Part model, mm, in its own coordinate system. Face numbers are marked on the shaded views. A direction names the side the tool comes from. Give positions to 0.01 mm unless a question says otherwise; leave off trailing zeros. Write each loop counter-clockwise with the first axis right and the second up, starting at its lowest first coordinate (ties: lowest second). Pieces come first, ordered by that corner, then holes. Notation, with made-up numbers: (-16.75, -14.5) - (30.25, -14.5) arc R4 ccw to (30.25, -7.5) - close; hole circle Ø7 at (-40, 28.25). An arc over 180 degrees is marked (long way). Answer in a Markdown table with one row per item. Add a question column.
1. Drop flat-ended pins along their axis: pin 1 Ø1.9 at (y, z) = (7.5, 1) entering from +X; pin 2 Ø4 at (y, z) = (-8.5, -30.5) entering from -X; pin 3 Ø4 at (x, z) = (11.43, -54.61) entering from +Y; pin 4 Ø6 at (x, y) = (23.5, -7.5) entering from +Z (3 decimals). Give the stop position or say it passes through.
2. Band-saw the part on B-B on z = -17.5. Write the cut outline in (x, y).
3. Probe line 1 along X through (y, z) = (2, -3.81); line 2 along X through (y, z) = (7.2, -54.61); line 3 along Z through (x, y) = (11, 3) (3 decimals). List the from-to ranges inside material, lowest first.
4. Which spindle directions (+Z, -Z, +X, -X, +Y, -Y) get a long thin tool onto all of the face, cutting with end or side? Do the marked faces 5, 6, 7, 8 and 9. Say none if no direction does.
5. Band-saw the part on D-D on x = 22. Write the cut outline in (y, z) (3 decimals).
6. Band-saw the part on A-A on x = 11.43. Write the cut outline in (y, z) (3 decimals), plus the area to 3 significant figures.
7. Pull direction Z, two halves, no side cores. Call the marked faces 1, 2, 3 and 4: released by +Z, released by -Z, zero draft, split by the parting line, or undercut.
8. Band-saw the part on C-C on y = -10.5. Write the cut outline in (x, z) (3 decimals).
```python
from build123d import *

# Parameters (mm, degrees)
SKETCH1_R           = 3.302
SKETCH1_R_2         = 2.615549664
BOSS_EXTRUDE1_DEPTH = 6.35
SKETCH2_W           = 30.48
SKETCH2_H           = 50.8
CUT_EXTRUDE1_DEPTH  = 3.81
CUT_EXTRUDE2_DEPTH  = 83.161835082
SKETCH13_R          = 2.615549664
BOSS_EXTRUDE7_DEPTH = 3.81
SKETCH15_W          = 7.62
SKETCH15_H          = 44.704
BOSS_EXTRUDE8_DEPTH = 21.59
SKETCH16_R          = 1.27
CUT_EXTRUDE3_DEPTH  = 81.375650193
FILLET1_R           = 2.54
CHAMFER2_SIZE       = 2.54


with BuildPart() as part:
    # Sketch1 → Boss-Extrude1 (new body)
    with BuildSketch(Plane(origin=(0, 0, 0), x_dir=(1, 0, 0), z_dir=(0, 1, 0))):
        Polygon((50.8, -0.508), (25.4, -5.588), (-25.4, -5.588), (-25.4, 64.262), (25.4, 64.262), (50.8, 59.182), align=None)
        with Locations(Location((0, 0, 0), (0, 0, 270))):
            Circle(SKETCH1_R, mode=Mode.SUBTRACT)
        with Locations(Location((0, 58.674, 0), (0, 0, 270))):
            Circle(SKETCH1_R, mode=Mode.SUBTRACT)
        with Locations(Location((11.43, 54.61, 0), (0, 0, 270))):
            Circle(SKETCH1_R_2, mode=Mode.SUBTRACT)
        with Locations(Location((-20.32, 54.61, 0), (0, 0, 270))):
            Circle(SKETCH1_R_2, mode=Mode.SUBTRACT)
        with Locations(Location((-20.32, 3.81, 0), (0, 0, 270))):
            Circle(SKETCH1_R_2, mode=Mode.SUBTRACT)
        with Locations(Location((11.43, 3.81, 0), (0, 0, 270))):
            Circle(SKETCH1_R_2, mode=Mode.SUBTRACT)
    extrude(amount=BOSS_EXTRUDE1_DEPTH)

    # Sketch2 → Cut-Extrude1 (cut)
    with BuildSketch(Plane(origin=(0, 6.35, 0), x_dir=(1, 0, 0), z_dir=(0, 1, 0))):
        with Locations((33.02, 29.337)):
            Rectangle(SKETCH2_W, SKETCH2_H)
    extrude(amount=-CUT_EXTRUDE1_DEPTH, mode=Mode.SUBTRACT)

    # Sketch3 → Cut-Extrude2 (cut, through all)
    with BuildSketch(Plane(origin=(0, 6.35, 0), x_dir=(1, 0, 0), z_dir=(0, 1, 0))):
        with BuildLine():
            Line((-15.24, 58.674), (-15.24, 51.689))
            Line((-15.24, 51.689), (5.08, 51.689))
            Line((5.08, 51.689), (5.08, 58.674))
            Line((5.08, 58.674), (3.302, 58.674))
            ThreePointArc((3.302, 58.674), (0, 55.372), (-3.302, 58.674))
            Line((-3.302, 58.674), (-15.24, 58.674))
        make_face()
        Polygon((-15.24, 51.689), (-25.4, 51.689), (-25.4, 6.985), (-15.24, 6.985), (5.08, 6.985), (17.78, 6.985), (17.78, 51.689), (5.08, 51.689), align=None)
        with BuildLine():
            Line((5.08, 6.985), (-15.24, 6.985))
            Line((-15.24, 6.985), (-15.24, 0))
            Line((-15.24, 0), (-3.302, 0))
            ThreePointArc((-3.302, 0), (0, 3.302), (3.302, 0))
            Line((3.302, 0), (5.08, 0))
            Line((5.08, 0), (5.08, 6.985))
        make_face()
    extrude(amount=-CUT_EXTRUDE2_DEPTH, mode=Mode.SUBTRACT)

    # Sketch13 → Boss-Extrude7 (add)
    # profile 1 of 2: a face of its own
    with BuildSketch(Plane(origin=(0, 6.35, 0), x_dir=(1, 0, 0), z_dir=(0, 1, 0))):
        with BuildLine():
            Line((-25.4, 64.262), (-25.4, 51.689))
            Line((-25.4, 51.689), (-15.24, 51.689))
            Line((-15.24, 51.689), (-15.24, 58.674))
            Line((-15.24, 58.674), (-3.302, 58.674))
            ThreePointArc((-3.302, 58.674), (0, 61.976), (3.302, 58.674))
            Line((3.302, 58.674), (5.08, 58.674))
            Line((5.08, 58.674), (5.08, 51.689))
            Line((5.08, 51.689), (17.78, 51.689))
            Line((17.78, 51.689), (17.78, 54.737))
            Line((17.78, 54.737), (25.4, 54.737))
            Line((25.4, 54.737), (25.4, 64.262))
            Line((25.4, 64.262), (-25.4, 64.262))
        make_face()
        with Locations(Location((-20.32, 54.61, 0), (0, 0, 270))):
            Circle(SKETCH13_R, mode=Mode.SUBTRACT)
        with Locations(Location((11.43, 54.61, 0), (0, 0, 270))):
            Circle(SKETCH13_R, mode=Mode.SUBTRACT)
    # profile 2 of 2: a face of its own
    with BuildSketch(Plane(origin=(0, 6.35, 0), x_dir=(1, 0, 0), z_dir=(0, 1, 0))):
        with BuildLine():
            Line((-15.24, 6.985), (-25.4, 6.985))
            Line((-25.4, 6.985), (-25.4, -5.588))
            Line((-25.4, -5.588), (25.4, -5.588))
            Line((25.4, -5.588), (25.4, 3.937))
            Line((25.4, 3.937), (17.78, 3.937))
            Line((17.78, 3.937), (17.78, 6.985))
            Line((17.78, 6.985), (5.08, 6.985))
            Line((5.08, 6.985), (5.08, 0))
            Line((5.08, 0), (3.302, 0))
            ThreePointArc((3.302, 0), (0, -3.302), (-3.302, 0))
            Line((-3.302, 0), (-15.24, 0))
            Line((-15.24, 0), (-15.24, 6.985))
        make_face()
        with Locations(Location((-20.32, 3.81, 0), (0, 0, 270))):
            Circle(SKETCH13_R, mode=Mode.SUBTRACT)
        with Locations(Location((11.43, 3.81, 0), (0, 0, 270))):
            Circle(SKETCH13_R, mode=Mode.SUBTRACT)
    extrude(amount=BOSS_EXTRUDE7_DEPTH)

    # Sketch15 → Boss-Extrude8 (add)
    with BuildSketch(Plane.XZ):
        with Locations((21.59, -29.337)):
            Rectangle(SKETCH15_W, SKETCH15_H)
    extrude(amount=BOSS_EXTRUDE8_DEPTH)

    # Sketch16 → Cut-Extrude3 (cut, through all)
    with BuildSketch(Plane.ZY.offset(-17.78)):
        with Locations((-44.323, -18.542)):
            Circle(SKETCH16_R)
        with Locations((-34.671, -18.542)):
            Circle(SKETCH16_R)
        with Locations((-24.003, -18.542)):
            Circle(SKETCH16_R)
        with Locations((-14.351, -18.542)):
            Circle(SKETCH16_R)
    extrude(amount=-CUT_EXTRUDE3_DEPTH, mode=Mode.SUBTRACT)

    # Fillet1
    # the kernel refuses this fillet: 2.54 mm, written as the material it adds along each edge
    with BuildSketch(Plane(origin=(-15.24, 0, -58.674), x_dir=(0, 0, 1), z_dir=(0, 1, 0))) as fillet1_piece_1:
        with BuildLine():
            CenterArc((FILLET1_R, FILLET1_R), FILLET1_R, 180, 90)
            Line((0, FILLET1_R), (0, 0))
            Line((0, 0), (FILLET1_R, 0))
        make_face()
    extrude(amount=10.16)
    with BuildSketch(Plane(origin=(5.08, 10.16, -58.674), x_dir=(-1, 0, 0), z_dir=(0, -1, 0))) as fillet1_piece_2:
        with BuildLine():
            CenterArc((2.54, -2.423005572), FILLET1_R, 107.457603124, 72.542396876)
            Line((0, -2.423005572), (0, 0))
            Line((0, 0), (1.778, 0))
        make_face()
    extrude(amount=10.16)
    with BuildSketch(Plane(origin=(5.08, 10.16, 0), x_dir=(0, 0, -1), z_dir=(0, -1, 0))) as fillet1_piece_3:
        with BuildLine():
            CenterArc((2.423005572, -2.54), FILLET1_R, 90, 72.542396876)
            Line((0, -1.778), (0, 0))
            Line((0, 0), (2.423005572, 0))
        make_face()
    extrude(amount=10.16)
    with BuildSketch(Plane(origin=(-15.24, 10.16, 0), x_dir=(1, 0, 0), z_dir=(0, -1, 0))) as fillet1_piece_4:
        with BuildLine():
            CenterArc((FILLET1_R, -FILLET1_R), FILLET1_R, 90, 90)
            Line((0, -FILLET1_R), (0, 0))
            Line((0, 0), (FILLET1_R, 0))
        make_face()
    extrude(amount=10.16)
    # the kernel refuses this fillet: 2.54 mm, written as the material it takes off along each edge
    with BuildSketch(Plane(origin=(-15.24, -6.35, -51.689), x_dir=(-1, 0, 0), z_dir=(0, 1, 0))) as fillet1_2_piece_1:
        with BuildLine():
            CenterArc((FILLET1_R, -FILLET1_R), FILLET1_R, 90, 90)
            Line((0, -FILLET1_R), (0, 0))
            Line((0, 0), (FILLET1_R, 0))
        make_face()
    extrude(amount=22.86, mode=Mode.SUBTRACT)
    with BuildSketch(Plane(origin=(5.08, 16.51, -51.689), x_dir=(0, 0, -1), z_dir=(0, -1, 0)), Plane(origin=(5.08, 16.51, -6.985), x_dir=(1, 0, 0), z_dir=(0, -1, 0)), Plane(origin=(-15.24, 16.51, -6.985), x_dir=(0, 0, 1), z_dir=(0, -1, 0))) as fillet1_2_piece_2:
        with BuildLine():
            CenterArc((FILLET1_R, FILLET1_R), FILLET1_R, 180, 90)
            Line((0, FILLET1_R), (0, 0))
            Line((0, 0), (FILLET1_R, 0))
        make_face()
    extrude(amount=22.86, mode=Mode.SUBTRACT)

    # Chamfer2
    chamfer2_edges = [part.edges().sort_by_distance(p)[0] for p in [
        (21.59, 0, -51.689),
        (25.4, 0, -29.337),
        (21.59, 0, -6.985),
    ]]
    chamfer(chamfer2_edges, length=CHAMFER2_SIZE)


solid = part.part
```
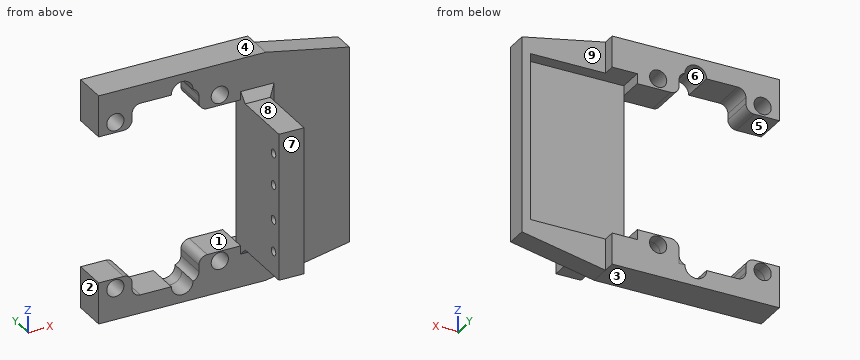
Values:
| question | item | result |
|---|---|---|
| 1 | pin 1 | stops at x = 25.4 |
| 1 | pin 2 | stops at x = 17.78 |
| 1 | pin 3 | passes through |
| 1 | pin 4 | stops at z = -6.985 |
| 2 | outline | (17.78, -21.59) - (25.4, -21.59) - (25.4, -2.54) - (27.94, 0) - (50.8, 0) - (50.8, 6.35) - (48.26, 6.35) - (48.26, 2.54) - (17.78, 2.54) - close |
| 3 | line 1 | x = -25.4 to -22.94, -17.7 to -15.24, 5.08 to 8.81, 14.05 to 50.8 |
| 3 | line 2 | x = -25.4 to -22.94, -17.7 to -15.24, 5.08 to 8.81, 14.05 to 17.78 |
| 3 | line 3 | z = -64.262 to -57.19, -52.03 to -51.689, -6.985 to -6.39, -1.23 to 5.588 |
| 4 | face 5 | -X, +Y, -Y |
| 4 | face 6 | +Y, -Y |
| 4 | face 7 | +Z, -Z, +X, -X, -Y |
| 4 | face 8 | +Z, +X, -X, -Y |
| 4 | face 9 | +Z, -Z, +X, +Y |
| 5 | outline | (-21.59, -51.689) - (-2.54, -51.689) - (0, -54.229) - (0, -64.262) - (10.16, -64.262) - (10.16, -54.737) - (2.54, -54.737) - (2.54, -3.937) - (10.16, -3.937) - (10.16, 5.588) - (0, 5.588) - (0, -4.445) - (-2.54, -6.985) - (-21.59, -6.985) - close; hole circle Ø2.54 at (-18.542, -44.323); hole circle Ø2.54 at (-18.542, -34.671); hole circle Ø2.54 at (-18.542, -24.003); hole circle Ø2.54 at (-18.542, -14.351) |
| 6 | outline | (0, -64.262) - (10.16, -64.262) - (10.16, -57.226) - (0, -57.226) - close; (0, -51.994) - (10.16, -51.994) - (10.16, -51.689) - (0, -51.689) - close; (0, -6.985) - (10.16, -6.985) - (10.16, -6.426) - (0, -6.426) - close; (0, -1.194) - (10.16, -1.194) - (10.16, 5.588) - (0, 5.588) - close |
| 6 | area | 149 mm² |
| 7 | face 1 | undercut |
| 7 | face 2 | zero draft |
| 7 | face 3 | released by -Z |
| 7 | face 4 | released by +Z |
| 8 | outline | (17.78, -51.689) - (25.4, -51.689) - (25.4, -6.985) - (17.78, -6.985) - close |
